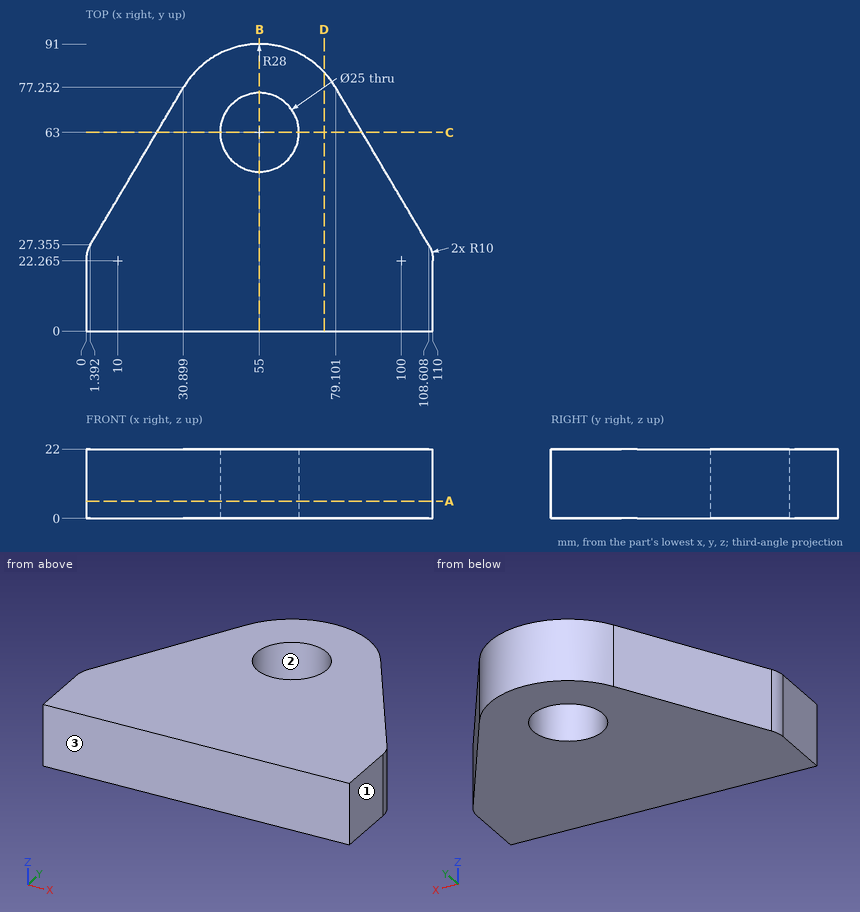
Source: three-view drawing plus pictorial views. Frame: mm from the lowest corner of the part. Give positions to 0.01 mm unless a question says otherwise; leave off trailing zeros. Order: outer loops, then holes, each group sorted by start corner. A loop starts at its lowest first (then second) coordinate and runs counter-clockwise, first axis right, second up. Notation, with made-up numbers: M 30,41 L 69,41 A10 cw 69,46 Z; hole C 35,62 d1. An arc over 180 degrees is marked long. One line per question, with ' | ' between items. Start each with the question number.
1. Pull-direction query (X, two-part tool) for the marked faces 1, 2 and 3; classes: released by +X, released by -X, zero draft, split by the parting line, or undercut.
2. First-contact query: pin 1 Ø5 at (y, z) = (57, 13) entering from +X (1 decimal); pin 2 Ø22.5 at (x, y) = (55, 63) entering from +Z; pin 3 Ø6 at (y, z) = (80, 19) entering from +X; pin 4 Ø1.5 at (y, z) = (41.5, 19.5) entering from +X. Flat tips, straight axial feed; report the tip coordinate or a pass-through.
3. Section query D-D (x = 75.5). Return the cut outline in (y, z).
4. Section query A-A (z = 5.5). Return the cut outline in (x, y) (1 decimal).
5. Section query B-B (x = 55). Return the cut outline in (y, z).
6. Material intervals for probe 1 along Y at (x, z) = (55, 13.75); probe 2 along Y at (x, z) = (53, 7); probe 3 along Y at (x, z) = (72.5, 12.75), sorted ascending. Write a range as [from, to].
7. Section query C-C (y = 63). Return the cut outline in (x, z), and give its area (3 significant figures).
Here are the results:
1) face 1: released by +X | face 2: undercut | face 3: zero draft
2) pin 1: x = 92.6 | pin 2: through | pin 3: x = 79.25 | pin 4: x = 100.69
3) outline: M 0,0 L 82.07,0 L 82.07,22 L 0,22 Z
4) outline: M 0,0 L 110,0 L 110,22.3 A10 ccw 108.6,27.4 L 79.1,77.3 A28 ccw 30.9,77.3 L 1.4,27.4 A10 ccw 0,22.3 Z; hole C 55,63 d25
5) outline: M 0,0 L 50.5,0 L 50.5,22 L 0,22 Z; M 75.5,0 L 91,0 L 91,22 L 75.5,22 Z
6) probe 1: [0, 50.5], [75.5, 91] | probe 2: [0, 50.66], [75.34, 90.93] | probe 3: [0, 84.86]
7) outline: M 22.47,0 L 42.5,0 L 42.5,22 L 22.47,22 Z; M 67.5,0 L 87.53,0 L 87.53,22 L 67.5,22 Z | area: 881 mm²
